from build123d import *

# Parameters (mm, degrees)
SKETCH3_W           = 13.5
SKETCH3_H           = 5
SKETCH3_W_2         = 10
SKETCH3_W_3         = 5
SKETCH3_H_2         = 23
BOSS_EXTRUDE1_DEPTH = 45
FILLET1_R           = 2
SKETCH5_R           = 2.1
CUT_EXTRUDE2_DEPTH  = 45
SKETCH6_R           = 2.1
CUT_EXTRUDE3_DEPTH  = 45
SKETCH7_W           = 8.210459319
SKETCH7_H           = 32.58724939
BOSS_EXTRUDE2_DEPTH = 5
SKETCH8_R           = 2.1
CUT_EXTRUDE5_DEPTH  = 45
BOSS_EXTRUDE3_DEPTH = 45


with BuildPart() as part:
    # Sketch3 → Boss-Extrude1 (new body)
    with BuildSketch(Plane.XY):
        with BuildLine():
            ThreePointArc((-5.06519953, 257.264696919), (-21.146881422, 239.197551787), (-25.551614771, 215.414352888))
            Line((-25.551614771, 215.414352888), (-30.551614771, 215.414352888))
            Line((-30.551614771, 215.414352888), (-30.551614771, 220.414352888))
            ThreePointArc((-30.551614771, 220.414352888), (-24.004098535, 245.112635185), (-5.06519953, 262.264696919))
            Line((-5.06519953, 262.264696919), (-5.06519953, 257.264696919))
        make_face()
        with Locations((1.68480047, 259.764696919)):
            Rectangle(SKETCH3_W, SKETCH3_H)
        with Locations((-35.551614771, 217.914352888)):
            Rectangle(SKETCH3_W_2, SKETCH3_H)
        with Locations((-28.051614771, 203.914352888)):
            Rectangle(SKETCH3_W_3, SKETCH3_H_2)
    extrude(amount=BOSS_EXTRUDE1_DEPTH)

    # Fillet1
    fillet1_edges = [part.edges().sort_by_distance(p)[0] for p in [
        (-40.551614771, 217.914352888, 0),
        (8.43480047, 259.764696919, 45),
        (8.43480047, 259.764696919, 0),
        (-40.551614771, 217.914352888, 45),
    ]]
    fillet(fillet1_edges, radius=FILLET1_R)

    # Sketch5 → Cut-Extrude2 (cut)
    with BuildSketch(Plane(origin=(0, 262.264696919, 0), x_dir=(1, 0, 0), z_dir=(0, 1, 0))):
        with Locations((0.24480047, -40)):
            Circle(SKETCH5_R)
        with Locations((0.24480047, -14.8)):
            Circle(SKETCH5_R)
    extrude(amount=-CUT_EXTRUDE2_DEPTH, mode=Mode.SUBTRACT)

    # Sketch6 → Cut-Extrude3 (cut)
    with BuildSketch(Plane(origin=(0, 220.414352888, 0), x_dir=(1, 0, 0), z_dir=(0, 1, 0))):
        with Locations((-35.551614771, -10)):
            Circle(SKETCH6_R)
        with Locations((-35.551614771, -35)):
            Circle(SKETCH6_R)
    extrude(amount=-CUT_EXTRUDE3_DEPTH, mode=Mode.SUBTRACT)

    # Sketch7 → Boss-Extrude2 (add)
    with BuildSketch(Plane(origin=(0, 262.264696919, 0), x_dir=(1, 0, 0), z_dir=(0, 1, 0))):
        with Locations((1.09445166, -26.923464517)):
            Rectangle(SKETCH7_W, SKETCH7_H)
    extrude(amount=-BOSS_EXTRUDE2_DEPTH)

    # Sketch8 → Cut-Extrude5 (cut)
    with BuildSketch(Plane(origin=(0, 262.264696919, 0), x_dir=(1, 0, 0), z_dir=(0, 1, 0))):
        with Locations((0.24480047, -5)):
            Circle(SKETCH8_R)
        with Locations((0.24480047, -30.2)):
            Circle(SKETCH8_R)
    extrude(amount=-CUT_EXTRUDE5_DEPTH, mode=Mode.SUBTRACT)

    # Sketch9 → Boss-Extrude3 (add, through all)
    with BuildSketch(Plane.XY.offset(45)):
        with BuildLine():
            ThreePointArc((-25.265361734, 225.859750777), (-25.456525287, 224.362535182), (-25.597369426, 222.859750777))
            Line((-25.597369426, 222.859750777), (-18.597369426, 222.859750777))
            Line((-18.597369426, 222.859750777), (-15.597369426, 222.859750777))
            Line((-15.597369426, 222.859750777), (-15.597369426, 247.859750777))
            ThreePointArc((-15.597369426, 247.859750777), (-17.156118075, 245.834377519), (-18.597369426, 243.72377838))
            Line((-18.597369426, 243.72377838), (-18.597369426, 225.859750777))
            Line((-18.597369426, 225.859750777), (-25.265361734, 225.859750777))
        make_face()
        Polygon((-15.597369426, 222.859750777), (-18.597369426, 222.859750777), (-25.551614771, 215.414352888), (-25.551614771, 212.414352888), align=None)
    extrude(amount=-BOSS_EXTRUDE3_DEPTH)


solid = part.part
Read the model definition and answer for the solid it produces. Units are mm, in the model's axes. A direction names the side the tool comes from. Round coordinates to 2 decimals unless told otherwise and drop trailing zeros. Write each loop counter-clockwise with the first axis right and the second up, starting at its lowest first coordinate (ties: lowest second). Pieces come first, ordered by that corner, then holes. Notation, with made-up numbers: (20, 19) - (70, 19) arc R16 cw to (70, 47) - close; hole circle Ø11 at (3, -35). An arc over 180 degrees is marked (long way). Use a Markdown table: item, result.
(1) The part is cut by section A-A (z = 30.2). Write down the section's boundary in (x, y), then the cut area to 3 significant figures.
Reported:
| item | result |
|---|---|
| outline | (-40.55, 215.41) - (-30.55, 215.41) - (-30.55, 192.41) - (-25.55, 192.41) - (-25.55, 212.41) - (-15.6, 222.86) - (-15.6, 247.86) arc R45 cw to (-5.07, 257.26) - (-1.86, 257.26) - (-1.86, 262.26) - (-5.07, 262.26) arc R45 ccw to (-30.55, 220.41) - (-40.55, 220.41) - close; (2.34, 257.26) - (8.43, 257.26) - (8.43, 262.26) - (2.34, 262.26) - close; hole (-25.6, 222.86) arc R45 ccw to (-25.55, 215.41) - (-18.6, 222.86) - close; hole (-25.27, 225.86) - (-18.6, 225.86) - (-18.6, 243.72) arc R45 ccw to start |
| area | 595 mm2 |
(2) Straight lines are drawn through the part: line 1 along X through (y, z) = (216, 10); line 2 along X through (y, z) = (218.3, 35); line 3 along Y through (x, z) = (-22, 12). For each, find the intervals that lie inside material, in ascending order. Write a range as [from, to].
Reported:
| item | result |
|---|---|
| line 1 | [-40.55, -37.65], [-33.45, -25.6], [-25, -22.13] |
| line 2 | [-40.55, -37.65], [-33.45, -25.72], [-22.86, -19.94] |
| line 3 | [216.14, 219.22], [222.86, 225.86], [237.35, 248.12] |
(3) Which of the six approach directions +Z, -Z, +X, -X, +Y, -Y give full straight-line access (tool end or side, diameter ignored) to faces 5 (the flat face through (-22.026, 219.189, 22.815)), 6 (the flat face through (8.435, 260, 22)), 7 (the flat face through (-15.597, 235, 23))?
Reported:
| item | result |
|---|---|
| face 5 | +Z, -Z |
| face 6 | +Z, -Z, +X, +Y, -Y |
| face 7 | +Z, -Z, +X, -Y |
(4) The part is cut by section D-D (y = 233). Write down the section's boundary in (x, z), then the cut area to 3 significant figures.
Reported:
| item | result |
|---|---|
| outline | (-29.13, 0) - (-23.63, 0) - (-23.63, 45) - (-29.13, 45) - close; (-18.6, 0) - (-15.6, 0) - (-15.6, 45) - (-18.6, 45) - close |
| area | 383 mm2 |
(5) The part is cut by section C-C (x = -24). Write down the section's boundary in (y, z), then the cut area to 3 significant figures.
Reported:
| item | result |
|---|---|
| outline | (214.04, 0) - (217.08, 0) - (217.08, 45) - (214.04, 45) - close; (222.86, 0) - (225.86, 0) - (225.86, 45) - (222.86, 45) - close; (231.77, 0) - (245.12, 0) - (245.12, 45) - (231.77, 45) - close |
| area | 872 mm2 |
(6) Each of these flat-tipped pins is pushed along its axis until it touches: pin 1 Ø8 at (y, z) = (251.5, 13.5) entering from -X; pin 2 Ø7.5 at (x, z) = (-21.5, 18) entering from -Y; pin 3 Ø7 at (y, z) = (209, 18.5) entering from -X; pin 4 Ø2.5 at (x, z) = (0.24, 30.2) entering from +Y. Where does it stop, or does it pass through?
Reported:
| item | result |
|---|---|
| pin 1 | x = -22.44 |
| pin 2 | y = 212.73 |
| pin 3 | x = -30.55 |
| pin 4 | through |
(7) The mould has two halves that part along Z. Classify faces 1 (the flat face through (-36, 220.414, 22)), 2 (the cylindrical face through (-33.55, 217.95, 9.37)), 3 (the cylindrical face through (-33.61, 217.95, 35.8)), 4 (the cylindrical face through (-39.98, 217.95, 0.6)): released by +Z, released by -Z, zero draft, split by the parting line, or undercut.
Reported:
| item | result |
|---|---|
| face 1 | zero draft |
| face 2 | undercut |
| face 3 | undercut |
| face 4 | released by -Z |
(8) The part is cut by section B-B (y = 219). Write down the section's boundary in (x, z), then the cut area to 3 significant figures.
Reported:
| item | result |
|---|---|
| outline | (-40.55, 2) arc R2 ccw to (-38.55, 0) - (-25.73, 0) - (-25.73, 45) - (-38.55, 45) arc R2 ccw to (-40.55, 43) - close; (-22.2, 0) - (-19.28, 0) - (-19.28, 45) - (-22.2, 45) - close; hole circle Ø4.2 at (-35.55, 10); hole circle Ø4.2 at (-35.55, 35) |
| area | 769 mm2 |
